Part model, mm, in its own coordinate system. A direction names the side the tool comes from. Give positions to 0.01 mm unless a question says otherwise; leave off trailing zeros. Order: outer loops, then holes, each group sorted by start corner. A loop starts at its lowest first (then second) coordinate and runs counter-clockwise, first axis right, second up. Notation, with made-up numbers: (69.5, 43.25) -> (122.5, 43.25) arc R25 ccw to (122.5, 78.25) -> close; hole circle Ø3 at (77.5, 17). An arc over 180 degrees is marked (long way). Write item = value, one per line. Start each with the question number.
(1) Which spindle directions (+Z, -Z, +X, -X, +Y, -Y) get a long thin tool onto all of the face, cutting with end or side? Do faces 1 (the flat face through (-0.86, -5.3, 5.67)), 2 (the flat face through (-0.97, -4.31, 11.25)), 3 (the flat face through (0, 4, 11)), 4 (the flat face through (0.97, 4.71, 5.93)), 5 (the flat face through (-0.86, 5.3, 5.67)). Say none if no direction does.
(2) Probe line 1 along Z through (x, y) = (1.7, 1.25); line 2 along Y through (x, z) = (0.1, 5.5); line 3 along Y through (x, z) = (-1.5, 6). List the from-to ranges inside material, lowest first. Write a range as from..to.
(3) Saw through at B-B, the plane z = 9.25. List the corners of the cut face in (x, y).
(4) Saw through at C-C, the plane x = 0.4. List the corners of the cut face in (y, z), then the cut area to 3 significant figures.
(5) Saw through at D-D, the plane y = 4.5. List the corners of the cut face in (x, z), then the cut area to 3 significant figures.
(6) Saw through at A-A, the plane y = -4. List the corners of the cut face in (x, z).
(7) Two-plate mould, pull along Z, no slides. Class faces 6 (the flat face through (0.83, -5.28, 5.67)), 7 (the flat face through (0, 4.6, 11.5)), 8 (the flat face through (-0.97, -4.71, 5.93)): pulls with the +Z half, pulls with the -Z half, needs draft (parallel to the pull), parting line crosses it, or undercut.
(8) Flat gauge pins, fed straight in: pin 1 (1 mm diameter, centred on x = 1.5, y = -2.5, fed in from +Z); pin 2 (1.5 mm diameter, centred on x = 0, z = 4, fed in from +Y); pin 3 (1 mm diameter, centred on x = 0.5, z = 10, fed in from +Y). Where does each tip first touch, or does it go through?
from build123d import *

# Parameters (mm, degrees)
BOSS_EXTRUDE1_DEPTH = 1
BOSS_EXTRUDE2_DEPTH = 11
BOSS_EXTRUDE4_DEPTH = 0.5


with BuildPart() as part:
    # Sketch1 → Boss-Extrude1 (new body)
    with BuildSketch(Plane.XY):
        Polygon((0, 4.801442841), (1.6875, 5.775721421), (1.96875, 5.288582131), (1.96875, -5.288582131), (1.6875, -5.775721421), (0, -4.801442841), (-1.6875, -5.775721421), (-1.96875, -5.288582131), (-1.96875, 5.288582131), (-1.6875, 5.775721421), align=None)
    extrude(amount=BOSS_EXTRUDE1_DEPTH)

    # Sketch2 → Boss-Extrude2 (add)
    with BuildSketch(Plane.XY):
        Polygon((0, -4.801442841), (0, -4.151923789), (-1.96875, -5.288582131), (-1.6875, -5.775721421), align=None)
        Polygon((1.96875, -5.288582131), (0, -4.151923789), (0, -4.801442841), (1.6875, -5.775721421), align=None)
        Polygon((-1.96875, 5.288582131), (0, 4.151923789), (0, 4.801442841), (-1.6875, 5.775721421), align=None)
        Polygon((0, 4.801442841), (0, 4.151923789), (1.96875, 5.288582131), (1.6875, 5.775721421), align=None)
    extrude(amount=BOSS_EXTRUDE2_DEPTH)

    # Sketch5 → Boss-Extrude4 (add)
    with BuildSketch(Plane.XY.offset(11)):
        Polygon((1.96875, -4.886658342), (0, -3.75), (0, -4.151923789), (1.96875, -5.288582131), align=None)
        Polygon((1.96875, -5.288582131), (0, -4.151923789), (0, -4.801442841), (1.6875, -5.775721421), align=None)
        Polygon((0, -4.801442841), (0, -4.151923789), (-1.96875, -5.288582131), (-1.6875, -5.775721421), align=None)
        Polygon((0, -4.151923789), (0, -3.75), (-1.96875, -4.886658342), (-1.96875, -5.288582131), align=None)
        Polygon((0, 4.801442841), (0, 4.151923789), (1.96875, 5.288582131), (1.6875, 5.775721421), align=None)
        Polygon((0, 4.151923789), (0, 3.75), (1.96875, 4.886658342), (1.96875, 5.288582131), align=None)
        Polygon((-1.96875, 5.288582131), (0, 4.151923789), (0, 4.801442841), (-1.6875, 5.775721421), align=None)
        Polygon((-1.96875, 4.886658342), (0, 3.75), (0, 4.151923789), (-1.96875, 5.288582131), align=None)
    extrude(amount=BOSS_EXTRUDE4_DEPTH)


solid = part.part
Results list:
q1.face_1 = +Z, -Z, -Y
q1.face_2 = +Z, -X
q1.face_3 = none
q1.face_4 = +X
q1.face_5 = +Z, -Z, +Y
q2.line_1 = 0..1
q2.line_2 = -4.86..-4.21, 4.21..4.86
q2.line_3 = -5.67..-5.02, 5.02..5.67
q3.outline = (-1.97, -5.29) -> (-1.69, -5.78) -> (0, -4.8) -> (1.69, -5.78) -> (1.97, -5.29) -> (0, -4.15) -> close; (-1.97, 5.29) -> (0, 4.15) -> (1.97, 5.29) -> (1.69, 5.78) -> (0, 4.8) -> (-1.69, 5.78) -> close
q4.outline = (-5.03, 0) -> (5.03, 0) -> (5.03, 11.5) -> (3.98, 11.5) -> (3.98, 11) -> (4.38, 11) -> (4.38, 1) -> (-4.38, 1) -> (-4.38, 11) -> (-3.98, 11) -> (-3.98, 11.5) -> (-5.03, 11.5) -> close
q4.area = 24.1 mm^2
q5.outline = (-1.97, 0) -> (1.97, 0) -> (1.97, 1) -> (0.6, 1) -> (0.6, 11) -> (1.3, 11) -> (1.3, 11.5) -> (-1.3, 11.5) -> (-1.3, 11) -> (-0.6, 11) -> (-0.6, 1) -> (-1.97, 1) -> close
q5.area = 17.3 mm^2
q6.outline = (-1.97, 0) -> (1.97, 0) -> (1.97, 1) -> (-1.97, 1) -> close; (-0.43, 11) -> (0.43, 11) -> (0.43, 11.5) -> (-0.43, 11.5) -> close
q7.face_6 = needs draft
q7.face_7 = pulls with the +Z half
q7.face_8 = undercut
q8.pin_1 = 1
q8.pin_2 = 5.23
q8.pin_3 = 5.38
